from build123d import *

# Parameters (mm, degrees)
SKETCH067_W     = 20
SKETCH067_H     = 25
SKETCH067_R     = 1.5
PAD024_DEPTH    = 3
SKETCH068_R     = 3
POCKET043_DEPTH = 2
SKETCH069_W     = 20
SKETCH069_H     = 4
PAD025_DEPTH    = 15
SKETCH085_R     = 1.65
SKETCH085_W     = 2
SKETCH085_H     = 7
POCKET052_DEPTH = 5


with BuildPart() as part:
    # Sketch067 → Pad024 (new body)
    with BuildSketch(Plane.XY):
        with Locations((-45, 2.5)):
            Rectangle(SKETCH067_W, SKETCH067_H)
        with Locations((-52.5, 5)):
            Circle(SKETCH067_R, mode=Mode.SUBTRACT)
        with Locations((-37.5, 5)):
            Circle(SKETCH067_R, mode=Mode.SUBTRACT)
        with Locations((-37.5, -5)):
            Circle(SKETCH067_R, mode=Mode.SUBTRACT)
        with Locations((-52.5, -5)):
            Circle(SKETCH067_R, mode=Mode.SUBTRACT)
    extrude(amount=PAD024_DEPTH)

    # Sketch068 (on Face10 of Pad024) → Pocket043 (cut)
    with BuildSketch(Plane.XY.offset(3)):
        with Locations((-52.5, 5)):
            Circle(SKETCH068_R)
        with Locations((-37.5, 5)):
            Circle(SKETCH068_R)
        with Locations((-37.5, -5)):
            Circle(SKETCH068_R)
        with Locations((-52.5, -5)):
            Circle(SKETCH068_R)
    extrude(amount=-POCKET043_DEPTH, mode=Mode.SUBTRACT)

    # Sketch069 (on Face5 of Pocket043) → Pad025 (join)
    with BuildSketch(Plane.XY.offset(3)):
        with Locations((-45, 13)):
            Rectangle(SKETCH069_W, SKETCH069_H)
    extrude(amount=PAD025_DEPTH)

    # Sketch085 (on Face25 of Pad025) → Pocket052 (cut)
    with BuildSketch(Plane.XZ.offset(-11)):
        with Locations((-40, 13)):
            Circle(SKETCH085_R)
        with Locations((-52, 8.5)):
            Rectangle(SKETCH085_W, SKETCH085_H)
        with Locations((-46, 8.5)):
            Rectangle(SKETCH085_W, SKETCH085_H)
    extrude(amount=-POCKET052_DEPTH, mode=Mode.SUBTRACT)


with BuildPart() as part_1:
    # Body008 placement: moved
    add(part.part.moved(Location((0, 0, 121))))


solid = part_1.part
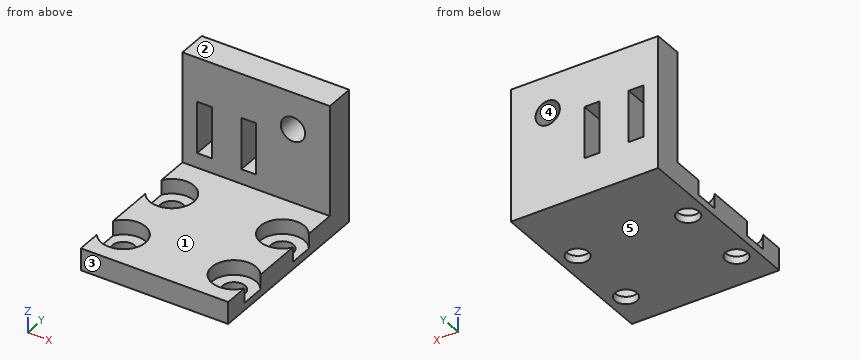
Design review of the part built by this model. Coordinates are the model's own, in mm. Face numbers are marked on the shaded views. A direction names the side the tool comes from. Coordinates: 2 decimals unless noted, no trailing zeros. Loops run counter-clockwise (first coordinate to the right, second up) from the corner with the lowest first, then second, coordinate; pieces in that order, holes last. Notation, with made-up numbers: M 4,57 L 16,57 A5 cw 16,61 Z; hole C 14,50.5 d4. An arc over 180 degrees is marked long. Answer as CSV lines item,"result".
Item 1: For probe 1 along Y at (x, z) = (-37.5, 123.55); probe 2 along Y at (x, z) = (-39.25, 126); probe 3 along Z at (x, y) = (-40.5, -0.5), list the stretches that pass through material, from the lowest coordinate up.
Answer list:
probe 1,"-10 to -8, -2 to 2, 8 to 15"
probe 2,"11 to 15"
probe 3,"121 to 124"
Item 2: For P1, Ø5, axis at x = -41, z = 127.5, coming from the -Y side; P2, Ø5, axis at x = -37.5, y = 5, coming from the +Z side, all flat-tipped, find the tip position at first contact; note any pin that passes through.
Answer list:
P1,"y = 11"
P2,"z = 122"
Item 3: Add section C-C on y = -5. State the section outline as (x, z) points.
Answer list:
outline,"M -55,121 L -54,121 L -54,122 L -55,122 Z; M -51,121 L -39,121 L -39,122 L -40.5,122 L -40.5,124 L -49.5,124 L -49.5,122 L -51,122 Z; M -36,121 L -35,121 L -35,122 L -36,122 Z"
Item 4: The part is to be moulded in two halves that separate along Z. For the marked faces 3, 4 and 5, say which applies: pulls with the +Z half, pulls with the -Z half, needs draft (parallel to the pull), parting line crosses it, or undercut.
Answer list:
face 3,"needs draft"
face 4,"undercut"
face 5,"pulls with the -Z half"
Item 5: Add section D-D on x = -46.5. State the section outline as (y, z) points, plus the area to 3 significant figures.
Answer list:
outline,"M -10,121 L 15,121 L 15,126 L 11,126 L 11,124 L -10,124 Z; M 11,133 L 15,133 L 15,139 L 11,139 Z"
area,"107 mm²"
Item 6: Add section B-B on x = -52.5. State the section outline as (y, z) points, plus the area to 3 significant figures.
Answer list:
outline,"M -10,121 L -6.5,121 L -6.5,122 L -8,122 L -8,124 L -10,124 Z; M -3.5,121 L 3.5,121 L 3.5,122 L 2,122 L 2,124 L -2,124 L -2,122 L -3.5,122 Z; M 6.5,121 L 15,121 L 15,126 L 11,126 L 11,124 L 8,124 L 8,122 L 6.5,122 Z; M 11,133 L 15,133 L 15,139 L 11,139 Z"
area,"77.0 mm²"
Item 7: Add section A-A on z = 128. State the section outline as (x, y) points.
Answer list:
outline,"M -55,11 L -53,11 L -53,15 L -55,15 Z; M -51,11 L -47,11 L -47,15 L -51,15 Z; M -45,11 L -35,11 L -35,15 L -45,15 Z"
Item 8: Machinability: for the marked faces 1 and 2, which of the approach directions +Z, -Z, +X, -X, +Y, -Y give a long, thin tool a straight path to every point of the face, cutting with its end or side? Answer none if there is none.
Answer list:
face 1,"+Z, +X, -X, -Y"
face 2,"+Z, +X, -X, +Y, -Y"
